Part model, mm, in its own coordinate system. Face numbers are marked on the shaded views. A direction names the side the tool comes from. Coordinates: 2 decimals unless noted, no trailing zeros. Order: outer loops, then holes, each group sorted by start corner. A loop starts at its lowest first (then second) coordinate and runs counter-clockwise, first axis right, second up. Notation, with made-up numbers: M -39,48.5 L -11,48.5 A11 ccw -11,58.5 Z; hole C 60.5,34.25 d11. An arc over 180 degrees is marked long. Write item = value, one per line. Start each with the question number.
Autodesk Inventor part; units mm, degrees
ref_plane "YZ Plane" through (0, 0, 0) normal (1, 0, 0) x (0, 1, 0)
ref_plane "XZ Plane" through (0, 0, 0) normal (0, 1, 0) x (-1, 0, 0)
ref_plane "XY Plane" through (0, 0, 0) normal (0, 0, 1) x (1, 0, 0)
sketch "スケッチ1" plane through (0, 0, 0) normal (0, 1, 0) x (-1, 0, 0)
  line L0 (0, 0) -> (40, 0)
  line L1 (40, 0) -> (40, -60)
  line L2 (40, -60) -> (0, -60)
  line L3 (0, -60) -> (0, 0)
  dimension "d0" = 40
  dimension "d1" = 60
extrude "押し出し1" add sketch "スケッチ1" along normal blind 2
sketch "スケッチ2" plane through (0, 0, 0) normal (1, 0, 0) x (0, 0, -1)
  line L0 (0, 2) -> (60, 2)
  line L1 (60, 2) -> (60, 30)
  line L2 (60, 30) -> (0, 30)
  line L3 (0, 30) -> (0, 2)
  point P0 (0, 0)
  dimension "d4" = 60
  dimension "d5" = 28
extrude "押し出し2" add sketch "スケッチ2" against normal blind 2
sketch "スケッチ5" plane through (0, 0, 0) normal (1, 0, 0) x (0, 0, -1)
  point P0 (0, 0)
sketch "スケッチ9" plane through (0, 0, 0) normal (0, -1, 0) x (1, 0, 0)
  point P0 (0, 0)
sketch "スケッチ11" plane through (0, 30, 0) normal (0, 1, 0) x (1, 0, 0)
  line L0 (0, 0) -> (-2, 0)
  line L1 (-2, 0) -> (-2, 60)
  line L2 (-2, 60) -> (0, 60)
  line L3 (0, 60) -> (0, 0)
extrude "押し出し6" cut sketch "スケッチ11" against normal blind 10
sketch "スケッチ12" plane through (0, 0, 0) normal (0, -1, 0) x (1, 0, 0)
  line L0 (0, -60) -> (0, 0)
  line L1 (0, -30) -> (-14, -30)
  dimension "d67" = 14
hole "穴4" at (-14, 0, -30) direction (0, 1, 0) diameter 12 end through all
sketch "スケッチ13" plane through (0, 0, 0) normal (0, -1, 0) x (1, 0, 0)
  line L0 (0, -60) -> (0, 0)
  line L1 (0, -30) -> (-20, -30)
  circle A0 centre (-20, -30) radius 15
  line L2 (-20, -30) -> (-20, -15)
  line L3 (-20, -30) -> (5.9808, -45)
  line L4 (-20, -30) -> (-149.9038, -105)
  point P0 (-7.0096, -37.5)
  point P1 (-32.9904, -37.5)
  dimension "d76" = 30
  dimension "d75" = 20
  dimension "d77" = 15
  dimension "d78" = 30
  dimension "d79" = 150
  dimension "d80" = 120
  dimension "d81" = 120
hole "穴5" at (-7.0096, 0, -37.5) at (-32.9904, 0, -37.5) at (-20, 0, -15) direction (0, 1, 0) diameter 3 end through all
properties part number "モーター固定"
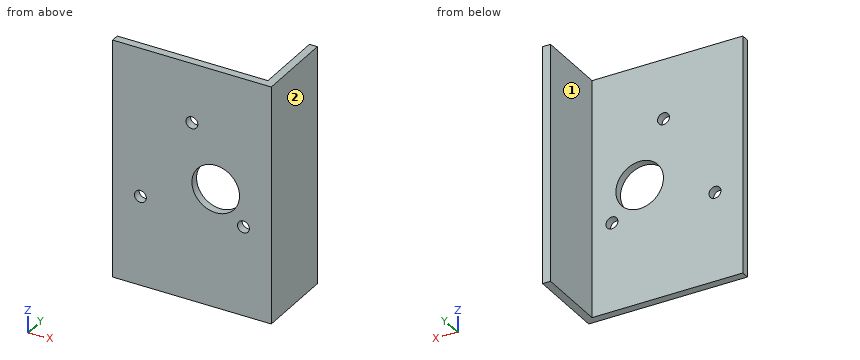
Item 1: Cut at A-A, the plane x = -14. Write the cut outline in (y, z).
Item 2: 3-axis set-ups, long thin cutter, end or side, ignore diameter. For the marked faces 1 and 2: which of +Z, -Z, +X, -X, +Y, -Y reach the whole face in a straight line?
Item 3: Cut at B-B, the plane z = -15. Write the cut outline in (x, y).
Item 4: Wall check: line 1 along X through (y, z) = (1.2, -15); line 2 along Z through (x, y) = (-14, 0.7); line 3 along X through (y, z) = (1.5, -30). Give the ranges that are in metal, low to high. Write a range as [from, to].
Item 5: Cut at C-C, the plane z = -9. Write the cut outline in (x, y).
Item 6: Cut at D-D, the plane y = 8.25. Write the cut outline in (x, z).
Item 7: Flat gauge pins, fed straight in: pin 1 (12 mm diameter, centred on y = 12, z = -41.5, fed in from -X); pin 2 (12 mm diameter, centred on x = -10, y = 7, fed in from -Z); pin 3 (1.8 mm diameter, centred on x = -20, z = -15, fed in from +Y). Where does each tip first touch, or does it go through?
Filled sheet:
q1.outline = M 0,-60 L 2,-60 L 2,-36 L 0,-36 Z; M 0,-24 L 2,-24 L 2,0 L 0,0 Z
q2.face_1 = +Z, -Z, -X, +Y
q2.face_2 = +Z, -Z, +X, +Y, -Y
q3.outline = M -40,0 L -21.5,0 L -21.5,2 L -40,2 Z; M -18.5,0 L 0,0 L 0,20 L -2,20 L -2,2 L -18.5,2 Z
q4.line_1 = [-40, -21.5], [-18.5, 0]
q4.line_2 = [-60, -36], [-24, 0]
q4.line_3 = [-40, -20], [-8, 0]
q5.outline = M -40,0 L 0,0 L 0,20 L -2,20 L -2,2 L -40,2 Z
q6.outline = M -2,-60 L 0,-60 L 0,0 L -2,0 Z
q7.pin_1 = -2
q7.pin_2 = -60
q7.pin_3 = through
